from build123d import *

# Parameters (mm, degrees)
SZKIC1_W                          = 850
SZKIC1_H                          = 1700
SZKIC1_W_2                        = 800
SZKIC1_H_2                        = 1650
SZKIC1_H_3                        = 25
SZKIC1_W_3                        = 25
WYCI_GNI_CIE_CIENKA_CIANKA1_DEPTH = 400
SZKIC2_R                          = 5
WYTNIJ_WYCI_GNI_CIE1_DEPTH        = 25
SZKIC4_R                          = 5
WYTNIJ_WYCI_GNI_CIE2_DEPTH        = 25
SZKIC6_R                          = 5
WYTNIJ_WYCI_GNI_CIE3_DEPTH        = 40


with BuildPart() as part:
    # Szkic1 → Wyciągnięcie-cienka ścianka1 (new body)
    # profile 1 of 5: a face of its own
    with BuildSketch(Plane.XY):
        with Locations((400, 825)):
            Rectangle(SZKIC1_W, SZKIC1_H)
        with Locations((400, 825)):
            Rectangle(SZKIC1_W_2, SZKIC1_H_2, mode=Mode.SUBTRACT)
    # profile 2 of 5: a face of its own
    with BuildSketch(Plane.XY):
        with Locations((400, 400)):
            Rectangle(SZKIC1_W_2, SZKIC1_H_3)
    # profile 3 of 5: a face of its own
    with BuildSketch(Plane.XY):
        with Locations((412.5, 825)):
            Rectangle(SZKIC1_W_3, SZKIC1_H_2)
    # profile 4 of 5: a face of its own
    with BuildSketch(Plane.XY):
        with Locations((400, 812.5)):
            Rectangle(SZKIC1_W_2, SZKIC1_H_3)
    # profile 5 of 5: a face of its own
    with BuildSketch(Plane.XY):
        with Locations((400, 1225)):
            Rectangle(SZKIC1_W_2, SZKIC1_H_3)
    extrude(amount=WYCI_GNI_CIE_CIENKA_CIANKA1_DEPTH)

    # Szkic2 → Wytnij-wyciągnięcie1 (cut)
    with BuildSketch(Plane(origin=(0, 825, 0), x_dir=(1, 0, 0), z_dir=(0, 1, 0))):
        with Locations(Location((70, -385.65, 0), (0, 0, 270))):
            Circle(SZKIC2_R)
        with Locations(Location((120, -385.65, 0), (0, 0, 270))):
            Circle(SZKIC2_R)
    extrude(amount=-WYTNIJ_WYCI_GNI_CIE1_DEPTH, mode=Mode.SUBTRACT)

    # Szkic4 → Wytnij-wyciągnięcie2 (cut)
    with BuildSketch(Plane(origin=(0, 825, 0), x_dir=(1, 0, 0), z_dir=(0, 1, 0))):
        with Locations(Location((730, -385.65, 0), (0, 0, 270))):
            Circle(SZKIC4_R)
        with Locations(Location((680, -385.65, 0), (0, 0, 270))):
            Circle(SZKIC4_R)
    extrude(amount=-WYTNIJ_WYCI_GNI_CIE2_DEPTH, mode=Mode.SUBTRACT)

    # Szkic6 → Wytnij-wyciągnięcie3 (cut)
    with BuildSketch(Plane.ZY.offset(25)):
        with Locations(Location((72.001673976, 1663, 0), (0, 0, 270))):
            Circle(SZKIC6_R)
        with Locations(Location((152.811673976, 1663, 0), (0, 0, 270))):
            Circle(SZKIC6_R)
    extrude(amount=-WYTNIJ_WYCI_GNI_CIE3_DEPTH, mode=Mode.SUBTRACT)


solid = part.part
Check sheet for the modelled part. Datum: model origin and axes. Units: mm. A direction names the side the tool comes from. Round coordinates to 2 decimals unless told otherwise and drop trailing zeros. Order: outer loops, then holes, each group sorted by start corner. A loop starts at its lowest first (then second) coordinate and runs counter-clockwise, first axis right, second up.
(1) Scan lines: probe 1 along Y at (x, z) = (481, 81); probe 2 along X at (y, z) = (818, 385); probe 3 along X at (y, z) = (1309.5, 289). Record each from-to range of solid material in increasing order.
(2) Cross-section at B-B, the plane x = 570. Enter the section's corners in (y, z), and give its area (3 significant figures).
(3) Cross-section at A-A, the plane y = 525.5. Enter the section's corners in (x, z).
(4) Draft check along X on faces 3 (the flat face through (394, -25, 197)), 4 (the flat face through (-25, 813, 197)), 5 (the flat face through (610, 800, 197)). Enter one of: pulls with the +X half, pulls with the -X half, needs draft (parallel to the pull), parting line crosses it, or undercut.
(5) Access from +Z, -Z, +X, -X, +Y, -Y to the whole of each face (thin tool, end or side, straight path). Record for faces 1 (the flat face through (394, 1675, 197)), 2 (the flat face through (800, 604, 197)).
(6) Cross-section at C-C, the plane z = 123.5. State how many separate pieces and enclosed holes the cut face has, and give its area (3 significant figures).
Check sheet entries:
1. probe 1: y = -25 to 0, 387.5 to 412.5, 800 to 825, 1212.5 to 1237.5, 1650 to 1675
1. probe 2: x = -25 to 65.04, 74.96 to 115.04, 124.96 to 675.04, 684.96 to 725.04, 734.96 to 825
1. probe 3: x = -25 to 0, 400 to 425, 800 to 825
2. outline: (-25, 0) - (0, 0) - (0, 400) - (-25, 400) - close; (387.5, 0) - (412.5, 0) - (412.5, 400) - (387.5, 400) - close; (800, 0) - (825, 0) - (825, 400) - (800, 400) - close; (1212.5, 0) - (1237.5, 0) - (1237.5, 400) - (1212.5, 400) - close; (1650, 0) - (1675, 0) - (1675, 400) - (1650, 400) - close
2. area: 50,000 mm2
3. outline: (-25, 0) - (0, 0) - (0, 400) - (-25, 400) - close; (400, 0) - (425, 0) - (425, 400) - (400, 400) - close; (800, 0) - (825, 0) - (825, 400) - (800, 400) - close
4. face 3: needs draft
4. face 4: pulls with the -X half
4. face 5: undercut
5. face 1: +Z, -Z, +X, -X, +Y
5. face 2: +Z, -Z
6. separate pieces: 1
6. enclosed holes: 8
6. area: 224,000 mm2
